from build123d import *

# Parameters (mm, degrees)
SKETCH_1_W      = 6
SKETCH_1_H      = 6
EXTRUDE_1_DEPTH = 2


with BuildPart() as part:
    # 草图1 → 凸台-拉伸1 (new body)
    with BuildSketch(Plane.XY):
        Rectangle(SKETCH_1_W, SKETCH_1_H)
    extrude(amount=EXTRUDE_1_DEPTH)

    # 草图3 → M3 螺纹孔1 (revolve, cut)
    with BuildSketch(Plane(origin=(0, 0, 2), x_dir=(0, -1, 0), z_dir=(1, 0, 0))):
        Polygon((0, 0), (0, 2), (1.525, 2), (1.25, 1.725), (1.25, 0.275), (1.525, 0), align=None)
    revolve(axis=Axis((0, 0, 8.35), (0, 0, -1)), mode=Mode.SUBTRACT)


solid = part.part
The listing builds one solid part. Answer for the finished solid, in the listing's coordinates (mm). Coordinates: 2 decimals unless noted, no trailing zeros. Write each loop counter-clockwise with the first axis right and the second up, starting at its lowest first coordinate (ties: lowest second). Pieces come first, ordered by that corner, then holes. Notation, with made-up numbers: M 87.5,-35.5 L 137.5,-35.5 A19 ccw 137.5,0.5 Z; hole C 15,-9.5 d2. An arc over 180 degrees is marked long. Use one line per item in the form item = value.
Item 1: Find section A-A, the plane y = 0. Give the vertices of the cut face in (x, z) (3 decimals), plus the area to 3 significant figures.
Model answer:
outline = M -3,0 L -1.525,0 L -1.25,0.275 L -1.25,1.725 L -1.525,2 L -3,2 Z; M 1.25,0.275 L 1.525,0 L 3,0 L 3,2 L 1.525,2 L 1.25,1.725 Z
area = 6.85 mm2
Item 2: Find the intervals of material crossed by probe 1 along X at (y, z) = (0, 1.15); probe 2 along X at (y, z) = (0.6, 0.9), in increasing order.
Model answer:
probe_1 = -3 to -1.25, 1.25 to 3
probe_2 = -3 to -1.1, 1.1 to 3
Item 3: Given P1, Ø3, axis at x = 0, y = 0, coming from the +Z side (3 decimals), flat-ended and moving along its own axis, determine where the tip first touches the part or whether it passes through.
Model answer:
P1 = 1.975
Item 4: Find section D-D, the plane z = 0.2. Give the vertices of the cut face in (x, y) (3 decimals).
Model answer:
outline = M -3,-3 L 3,-3 L 3,3 L -3,3 Z; hole C 0,0 d2.65
Item 5: The mould has two halves that part along X. Classify faces 1 (the face through (-1.4, 1.4, 0)), 2 (the face through (3, 0, 1)), 3 (the face through (1.22, 0.27, 1.01)), 4 (the face through (-3, 0, 1)): released by +X, released by -X, zero draft, split by the parting line, or undercut.
Model answer:
face_1 = zero draft
face_2 = released by +X
face_3 = undercut
face_4 = released by -X
Item 6: Find section C-C, the plane z = 1. Give the vertices of the cut face in (x, y).
Model answer:
outline = M -3,-3 L 3,-3 L 3,3 L -3,3 Z; hole C 0,0 d2.5
